Input: part model. Units: mm. Frame: model coordinates. A direction names the side the tool comes from. Give positions to 0.01 mm unless a question says otherwise; leave off trailing zeros. Loops run counter-clockwise (first coordinate to the right, second up) from the corner with the lowest first, then second, coordinate; pieces in that order, holes last. Notation, with made-up numbers: (46.25, -25.75) -> (50.25, -25.75) arc R29 ccw to (50.25, 12.25) -> close; hole circle Ø4 at (8, 16.25). An arc over 180 degrees is marked (long way). Answer as a JSON object with one key per item and string values.
```python
from build123d import *

# Parameters (mm, degrees)
SKETCH1_W           = 26
SKETCH1_H           = 15
SKETCH1_R           = 2
BOSS_EXTRUDE1_DEPTH = 7
CUT_EXTRUDE1_DEPTH  = 16
FILLET1_R           = 1


with BuildPart() as part:
    # Sketch1 → Boss-Extrude1 (new body)
    with BuildSketch(Plane.XY):
        with Locations((13, 7.5)):
            Rectangle(SKETCH1_W, SKETCH1_H)
        with Locations((13, 7.5)):
            Circle(SKETCH1_R, mode=Mode.SUBTRACT)
    extrude(amount=BOSS_EXTRUDE1_DEPTH)

    # Sketch2 → Cut-Extrude1 (cut, through all)
    with BuildSketch(Plane(origin=(0, 15, 0), x_dir=(1, 0, 0), z_dir=(0, 1, 0))):
        with BuildLine():
            Line((2.100252532, -7), (5.342893219, -3.757359313))
            ThreePointArc((5.342893219, -3.757359313), (6.05, -3.464466094), (6.757106781, -3.757359313))
            Line((6.757106781, -3.757359313), (9.999747468, -7))
            Line((9.999747468, -7), (2.100252532, -7))
        make_face()
        with BuildLine():
            Line((16.000252532, -7), (19.242893219, -3.757359313))
            ThreePointArc((19.242893219, -3.757359313), (19.95, -3.464466094), (20.657106781, -3.757359313))
            Line((20.657106781, -3.757359313), (23.899747468, -7))
            Line((23.899747468, -7), (16.000252532, -7))
        make_face()
    extrude(amount=-CUT_EXTRUDE1_DEPTH, mode=Mode.SUBTRACT)

    # Fillet1
    fillet1_edges = [part.edges().sort_by_distance(p)[0] for p in [
        (26, 7.5, 7),
        (9.999747468, 7.5, 7),
        (2.100252532, 7.5, 7),
        (23.899747468, 7.5, 7),
        (16.000252532, 7.5, 7),
        (0, 7.5, 7),
    ]]
    fillet(fillet1_edges, radius=FILLET1_R)


solid = part.part
```
Q1. Access query for faces 4 (the flat face through (8, 8, 5)), 5 (the flat face through (13, 15, 3)). Directions: +Z, -Z, +X, -X, +Y, -Y. A direction counts if a zero-diameter tool reaches every point of the face in a straight line with its end or side. Return the directions, or none.
Evaluation:
{"face 4": "+Z, +Y, -Y", "face 5": "+Z, -Z, +X, -X, +Y"}
Q2. Section A-A, the plane y = 7.5. Return the cut outline in (x, z).
Evaluation:
{"outline": "(0, 0) -> (11, 0) -> (11, 7) -> (10.41, 7) arc R1 ccw to (9.71, 6.71) -> (6.76, 3.76) arc R1 cw to (5.34, 3.76) -> (2.39, 6.71) arc R1 ccw to (1.69, 7) -> (1, 7) arc R1 ccw to (0, 6) -> close; (15, 0) -> (26, 0) -> (26, 6) arc R1 ccw to (25, 7) -> (24.31, 7) arc R1 ccw to (23.61, 6.71) -> (20.66, 3.76) arc R1 cw to (19.24, 3.76) -> (16.29, 6.71) arc R1 ccw to (15.59, 7) -> (15, 7) -> close"}
Q3. Draft query along X for faces 1 (the cylindrical face through (25.715, 7.605, 6.699)), 2 (the cylindrical face through (11.526, 8.852, 3.451)), 3 (the flat face through (11.8, 9.3, 7)). Return one class per face: +X half, -X half, draft (parallel to the pull), parting line (faces both ways), or undercut.
Evaluation:
{"face 1": "+X half", "face 2": "undercut", "face 3": "draft"}
Q4. Section B-B, the plane z = 5.5. Return the cut outline in (x, y).
Evaluation:
{"outline": "(0, 0) -> (3.6, 0) -> (3.6, 15) -> (0, 15) -> close; (8.5, 0) -> (17.5, 0) -> (17.5, 15) -> (8.5, 15) -> close; (22.4, 0) -> (26, 0) -> (26, 15) -> (22.4, 15) -> close; hole circle Ø4 at (13, 7.5)"}
Q5. Section D-D, the plane y = 1.75. Return the cut outline in (x, z).
Evaluation:
{"outline": "(0, 0) -> (26, 0) -> (26, 6) arc R1 ccw to (25, 7) -> (24.31, 7) arc R1 ccw to (23.61, 6.71) -> (20.66, 3.76) arc R1 cw to (19.24, 3.76) -> (16.29, 6.71) arc R1 ccw to (15.59, 7) -> (10.41, 7) arc R1 ccw to (9.71, 6.71) -> (6.76, 3.76) arc R1 cw to (5.34, 3.76) -> (2.39, 6.71) arc R1 ccw to (1.69, 7) -> (1, 7) arc R1 ccw to (0, 6) -> close"}
Q6. Ray query, line 1 along Y through (x, z) = (13, 2.25); line 2 along Z through (x, y) = (17.5, 9.25); line 3 along X through (y, z) = (7.75, 0.5). Return the intervals inside material, ascending.
Evaluation:
{"line 1": "y = 0 to 5.5, 9.5 to 15", "line 2": "z = 0 to 5.5", "line 3": "x = 0 to 11.02, 14.98 to 26"}
Q7. Section C-C, the plane x = 13. Return the cut outline in (y, z).
Evaluation:
{"outline": "(0, 0) -> (5.5, 0) -> (5.5, 7) -> (0, 7) -> close; (9.5, 0) -> (15, 0) -> (15, 7) -> (9.5, 7) -> close"}
